Answer from the drawing. Dimensions are ordinates in mm from the lowest x, y and z of the part. A direction names the side the tool comes from. Give positions to 0.01 mm unless a question says otherwise; leave off trailing zeros. Loops run counter-clockwise (first coordinate to the right, second up) from the corner with the lowest first, then second, coordinate; pieces in that order, holes last. Notation, with made-up numbers: (43.25, -37) - (101.25, -37) arc R25 cw to (101.25, -6) - close; hole circle Ø7 at (0.5, 5). An arc over 180 degrees is marked (long way). One line per question, with ' | ' between items. Start each with the question number.
1. Each of these flat-tipped pins is pushed along its axis until it touches: pin 1 (2 mm diameter, centred on x = 31, z = 13, fed in from +Y); pin 2 (10 mm diameter, centred on x = 50.5, y = 27, fed in from +Z); pin 3 (0.8 mm diameter, centred on x = 71, y = 0.5, fed in from +Z). Where does it stop, or does it pass through?
2. For a pull along X with two mould halves and no side action, classify the marked faces 1, 2, 3 and 4 as released by +X, released by -X, zero draft, split by the parting line, or undercut.
3. Section A-A (z = 17) is taken. Determine the outline of the cut face in (x, y).
4. Which of the six approach directions +Z, -Z, +X, -X, +Y, -Y give full straight-line access (tool end or side, diameter ignored) to the marked faces 5 and 6?
5. Section B-B (x = 29) is taken. Determine the outline of the cut face in (y, z).
6. Section D-D (z = 12.25) is taken. Determine the outline of the cut face in (x, y).
7. Find the intervals of material crossed by line 1 (Y direction, x = 68, z = 3.5); line 2 (X direction, y = 10.5, z = 11.25); line 3 (Y direction, x = 71, z = 13.5), in increasing order.
8. Section C-C (y = 36.5) is taken. Determine the outline of the cut face in (x, z), plus the area to 3 significant figures.
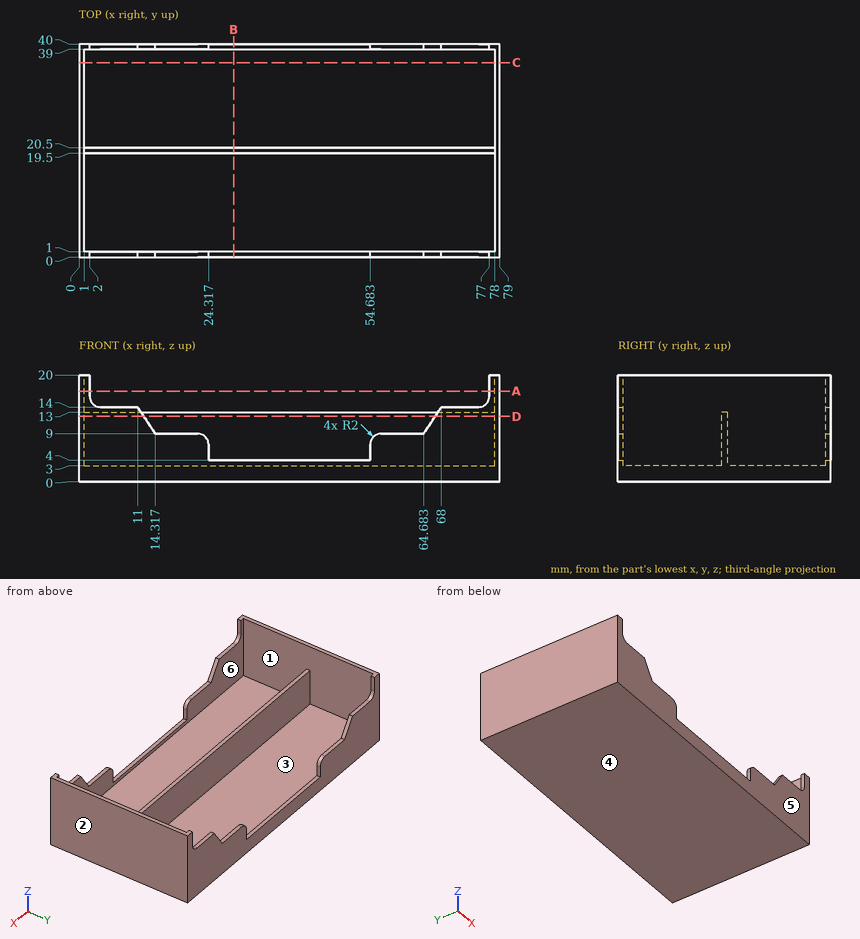
Conclusion:
1) pin 1: y = 20.5 | pin 2: z = 3 | pin 3: z = 14
2) face 1: undercut | face 2: released by +X | face 3: undercut | face 4: zero draft
3) outline: (0, 0) - (2, 0) - (2, 1) - (1, 1) - (1, 39) - (2, 39) - (2, 40) - (0, 40) - close; (77, 0) - (79, 0) - (79, 40) - (77, 40) - (77, 39) - (78, 39) - (78, 1) - (77, 1) - close
4) face 5: +Z, -Z, +X, -X, -Y | face 6: +Z
5) outline: (0, 0) - (40, 0) - (40, 4) - (39, 4) - (39, 3) - (20.5, 3) - (20.5, 13) - (19.5, 13) - (19.5, 3) - (1, 3) - (1, 4) - (0, 4) - close
6) outline: (0, 0) - (12.16, 0) - (12.16, 1) - (1, 1) - (1, 19.5) - (78, 19.5) - (78, 1) - (66.84, 1) - (66.84, 0) - (79, 0) - (79, 40) - (66.84, 40) - (66.84, 39) - (78, 39) - (78, 20.5) - (1, 20.5) - (1, 39) - (12.16, 39) - (12.16, 40) - (0, 40) - close
7) line 1: 0 to 1, 19.5 to 20.5, 39 to 40 | line 2: 0 to 1, 78 to 79 | line 3: 0 to 1, 39 to 40
8) outline: (0, 0) - (79, 0) - (79, 20) - (78, 20) - (78, 3) - (1, 3) - (1, 20) - (0, 20) - close | area: 271 mm²
